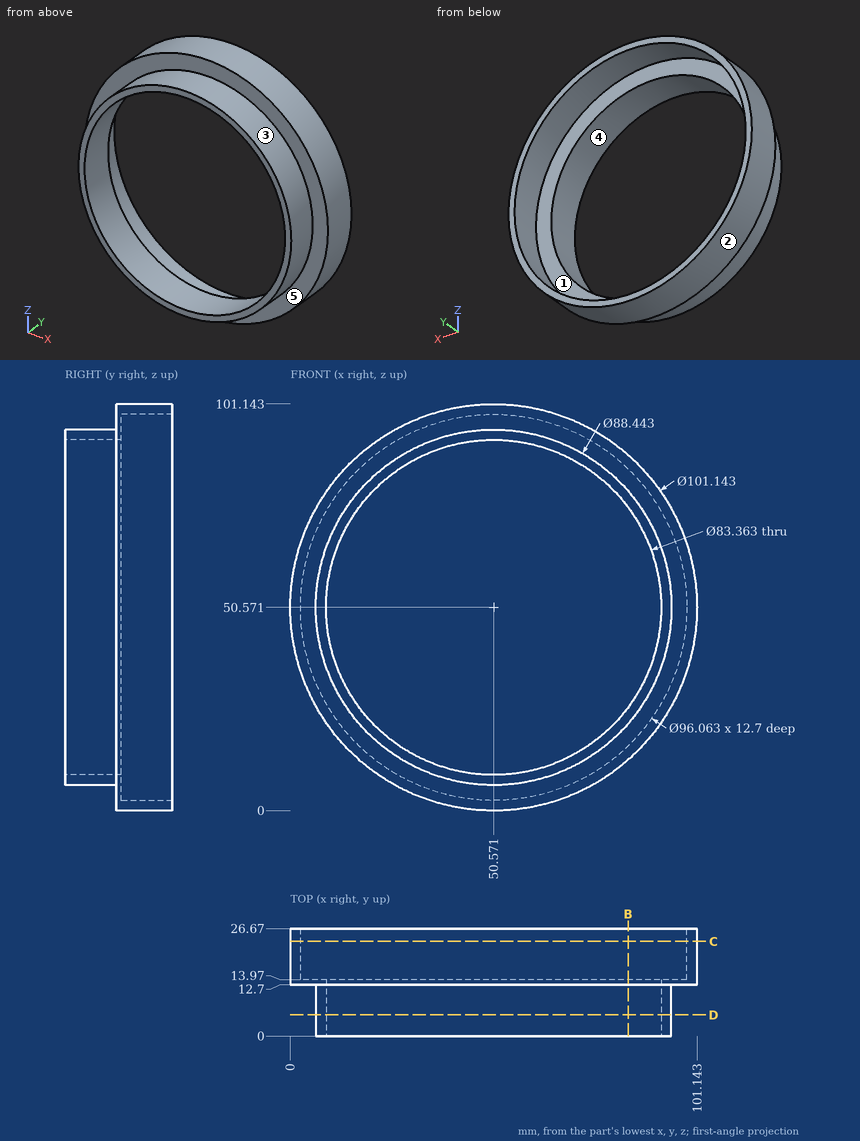
The drawing under review shows one solid part. Ordinate dimensions are in mm from its lowest x, y, z. A direction names the side the tool comes from. Coordinates: 2 decimals unless noted, no trailing zeros. Loops run counter-clockwise (first coordinate to the right, second up) from the corner with the lowest first, then second, coordinate; pieces in that order, holes last.
Item 1: Clearance check with flat-ended pins moving along their axes: pin 1 (8 mm diameter, centred on x = 72, y = 11.5, fed in from +Z); pin 2 (2 mm diameter, centred on y = 22, z = 82, fed in from -X); pin 3 (10 mm diameter, centred on y = 12, z = 10.5, fed in from +X). State where each tip first meets the part, or that it passes through.
Completed:
pin 1: stops at z = 97.98
pin 2: stops at x = 10.18
pin 3: stops at x = 86.96
Item 2: Draft analysis for pull direction Z (two halves, no side actions). For the marked faces 3, 4 and 5, state which applies: pulls with the +Z half, pulls with the -Z half, needs draft (parallel to the pull), parting line crosses it, or undercut.
Completed:
face 3: parting line crosses it
face 4: undercut
face 5: needs draft
Item 3: Add section C-C (y = 23.5). Write out the cut boundary in (x, z).
Completed:
outline: circle Ø101.14 at (50.57, 50.57); hole circle Ø96.06 at (50.57, 50.57)
Item 4: Add section D-D (y = 5.25). Write out the cut boundary in (x, z).
Completed:
outline: circle Ø88.44 at (50.57, 50.57); hole circle Ø83.36 at (50.57, 50.57)
Item 5: Add section B-B (x = 84). Write out the cut boundary in (y, z) (1 decimal), and give its area (3 significant figures).
Completed:
outline: (0, 21.6) - (12.7, 21.6) - (12.7, 12.6) - (26.7, 12.6) - (26.7, 16.1) - (14, 16.1) - (14, 25.7) - (0, 25.7) - close; (0, 75.5) - (14, 75.5) - (14, 85.1) - (26.7, 85.1) - (26.7, 88.5) - (12.7, 88.5) - (12.7, 79.5) - (0, 79.5) - close
area: 224 mm2
Item 6: For the marked faces 1 and 2, list the 3-axis set-ups (+Z, -Z, +X, -X, +Y, -Y) from which the entire face can be reached by the end or side of a thin tool; tool diameter is ignored.
Completed:
face 1: +Y
face 2: +Y, -Y
Item 7: Wall thickness on L1, parallel to X at y = 22, z = 25.5; L2, parallel to Z at x = 14.5, y = 20.75 (1 decimal); L3, parallel to Z at x = 81, y = 11 (1 decimal): over which ranges is each line inside the solid? List them lowest first.
Completed:
L1: x = 6.65 to 9.6, 91.54 to 94.49
L2: z = 15.1 to 18.9, 82.3 to 86
L3: z = 18.5 to 22.1, 79.1 to 82.7
